Build history of the part. All positions in model axes, mm. A direction names the side the tool comes from. Round coordinates to 2 decimals unless told otherwise and drop trailing zeros. Loops run counter-clockwise (first coordinate to the right, second up) from the corner with the lowest first, then second, coordinate; pieces in that order, holes last.
from build123d import *

# Parameters (mm, degrees)
F0_R     = 13.160254
F0_R_2   = 1.5
F0_R_3   = 4
F1_DEPTH = 3
F2_R     = 6
F2_R_2   = 4
F3_DEPTH = 7
F4_R     = 4
F5_DEPTH = 25


with BuildPart() as f1:
    # F0 (on Front) → F1 (new body)
    with BuildSketch(Plane.XZ):
        Circle(F0_R)
        with Locations((-6.056582, -6.190139)):
            Circle(F0_R_2, mode=Mode.SUBTRACT)
        with Locations((8.389108, -2.150084)):
            Circle(F0_R_2, mode=Mode.SUBTRACT)
        with Locations((-2.332527, 8.340223)):
            Circle(F0_R_2, mode=Mode.SUBTRACT)
        Circle(F0_R_3, mode=Mode.SUBTRACT)
    extrude(amount=F1_DEPTH)

    # F2 (on face) → F3 (join)
    with BuildSketch(Plane.XZ.offset(3)):
        Circle(F2_R)
        Circle(F2_R_2, mode=Mode.SUBTRACT)
    extrude(amount=F3_DEPTH)

    # F4 (on face) → F5 (cut)
    with BuildSketch(Plane.XZ.offset(3)):
        with Locations((-2.332527, 8.340223)):
            Circle(F4_R)
        with Locations((8.389108, -2.150084)):
            Circle(F4_R)
        with Locations((-6.056582, -6.190139)):
            Circle(F4_R)
    extrude(amount=F5_DEPTH, mode=Mode.SUBTRACT)


solid = f1.part
(1) Which spindle directions (+Z, -Z, +X, -X, +Y, -Y) get a long thin tool onto all of the face, cutting with end or side? Do faces 1 (the face through (1.57, -6.45, -5.79)), 2 (the face through (6, -3, 0)), 3 (the face through (4.524, -6.451, -1.122)). Say none if no direction does.
Responses:
face 1: -Z, -Y
face 2: -Y
face 3: +X, -Y
(2) Slice it at D-D on z = 8. List the corners of the cut face in (x, y).
Responses:
outline: (-10.45, -3) - (-3.79, -3) - (-3.79, 0) - (-10.45, 0) - close; (-0.87, -3) - (10.45, -3) - (10.45, 0) - (-0.87, 0) - close
(3) Pin check, flat tips, straight feed: P1, Ø1, axis at x = 4, y = -9, coming from the +Z side; P2, Ø5, axis at y = -1.5, z = 8, coming from the -X side; P3, Ø4, axis at x = -6.06, z = -6.19, coming from the -Y side. Stop position of each tip, or through.
Responses:
P1: stops at z = 4.87
P2: stops at x = -11.96
P3: stops at y = -3
(4) Slice it at B-B on z = 0. List the corners of the cut face in (x, y), plus the area to 3 significant figures.
Responses:
outline: (-13.16, -3) - (-6, -3) - (-6, -10) - (-4, -10) - (-4, 0) - (-13.16, 0) - close; (4, -10) - (5.02, -10) - (5.02, -3) - (13.16, -3) - (13.16, 0) - (4, 0) - close
area: 76.1 mm2
(5) Probe line 1 (X direction, y = -0.25, z = -1.75); line 2 (X direction, y = -2.75, z = -1.5); line 3 (Y direction, x = -1, z = -11.25). List the from-to ranges inside material, lowest first.
Responses:
line 1: x = -13.04 to -3.6, 3.6 to 6.94, 9.83 to 13.04
line 2: x = -13.07 to -3.71, 3.71 to 7.04, 9.74 to 13.07
line 3: y = -3 to 0
(6) Pull direction Z, two halves, no side cores. Call faces 4 (the face through (-1.526, -1.479, 9.605)), 5 (the face through (-5.8, -6.45, 1.54)), 6 (the face through (-3.23, -6.45, -3.36)), 7 (the face through (4.234, -6.451, 4.251)): +Z half, -Z half, draft (parallel to the pull), parting line (faces both ways), or undercut.
Responses:
face 4: undercut
face 5: parting line
face 6: -Z half
face 7: +Z half
(7) Slice it at A-A on y = -7. List the corners of the cut face in (x, z).
Responses:
outline: (-5.57, -2.22) arc R4 cw to (-2.1, -5.62) arc R6 ccw to (4.71, -3.72) arc R4 cw to (5.92, 0.99) arc R6 ccw to (0.87, 5.94) arc R4 cw to (-3.82, 4.63) arc R6 ccw to start; hole circle Ø8 at (0, 0)
(8) Slice it at C-C on x = 1.5. List the corners of the cut face in (y, z).
Responses:
outline: (-10, -5.81) - (-3, -5.81) - (-3, -13.07) - (0, -13.07) - (0, -3.71) - (-10, -3.71) - close; (-10, 3.71) - (0, 3.71) - (0, 13.07) - (-3, 13.07) - (-3, 5.81) - (-10, 5.81) - close
